```python
from build123d import *

# Parameters (mm, degrees)
SKETCH1_W           = 70
SKETCH1_H           = 25
SKETCH1_R           = 1.6
BOSS_EXTRUDE2_DEPTH = 10
SKETCH2_W           = 70
SKETCH2_H           = 5
BOSS_EXTRUDE3_DEPTH = 50
SKETCH3_R           = 3.5
CUT_EXTRUDE1_DEPTH  = 5
FILLET1_R           = 4
FILLET2_R           = 10
SKETCH4_R           = 1.6
CUT_EXTRUDE2_DEPTH  = 96.524865873


with BuildPart() as part:
    # Sketch1 → Boss-Extrude2 (new body)
    with BuildSketch(Plane(origin=(0, 0, 0), x_dir=(1, 0, 0), z_dir=(0, 1, 0))):
        with Locations((35, 12.5)):
            Rectangle(SKETCH1_W, SKETCH1_H)
        with Locations(Location((20, 15, 0), (0, 0, 270))):
            Circle(SKETCH1_R, mode=Mode.SUBTRACT)
        with Locations(Location((50, 15, 0), (0, 0, 270))):
            Circle(SKETCH1_R, mode=Mode.SUBTRACT)
    extrude(amount=BOSS_EXTRUDE2_DEPTH)

    # Sketch2 → Boss-Extrude3 (add)
    with BuildSketch(Plane(origin=(0, 10, 0), x_dir=(1, 0, 0), z_dir=(0, 1, 0))):
        with Locations((35, 2.5)):
            Rectangle(SKETCH2_W, SKETCH2_H)
    extrude(amount=BOSS_EXTRUDE3_DEPTH)

    # Sketch3 → Cut-Extrude1 (cut)
    with BuildSketch(Plane(origin=(0, 10, 0), x_dir=(1, 0, 0), z_dir=(0, 1, 0))):
        with Locations(Location((20, 15, 0), (0, 0, 270))):
            Circle(SKETCH3_R)
        with Locations(Location((50, 15, 0), (0, 0, 270))):
            Circle(SKETCH3_R)
    extrude(amount=-CUT_EXTRUDE1_DEPTH, mode=Mode.SUBTRACT)

    # Fillet1
    fillet1_edges = [part.edges().sort_by_distance(p)[0] for p in [
        (35, 10, -5),
    ]]
    fillet(fillet1_edges, radius=FILLET1_R)

    # Fillet2
    fillet2_edges = [part.edges().sort_by_distance(p)[0] for p in [
        (0, 60, -2.5),
        (70, 60, -2.5),
        (0, 5, -25),
        (70, 5, -25),
    ]]
    fillet(fillet2_edges, radius=FILLET2_R)

    # Sketch4 → Cut-Extrude2 (cut, through all)
    with BuildSketch(Plane.XY):
        with Locations((10, 50)):
            Circle(SKETCH4_R)
        with Locations((18, 50)):
            Circle(SKETCH4_R)
        with Locations((52, 50)):
            Circle(SKETCH4_R)
        with Locations((60, 50)):
            Circle(SKETCH4_R)
    extrude(amount=-CUT_EXTRUDE2_DEPTH, mode=Mode.SUBTRACT)


solid = part.part
```
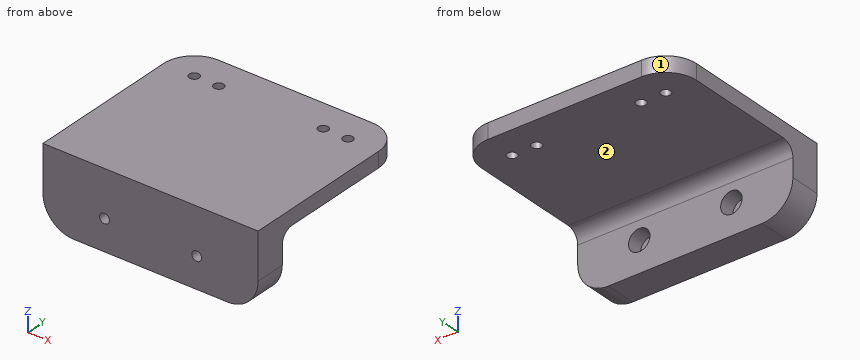
For this review, take the finished solid that the model builds, in its own axes (mm). Face numbers are marked on the shaded views. A direction names the side the tool comes from. Give positions to 0.01 mm unless a question says otherwise; leave off trailing zeros. Write each loop counter-clockwise with the first axis right and the second up, starting at its lowest first coordinate (ties: lowest second). Pieces come first, ordered by that corner, then holes.
Item 1: Wall thickness on probe 1 along X at (y, z) = (8.85, -15); probe 2 along X at (y, z) = (2.25, -15); probe 3 along Y at (x, z) = (10, -3.55): over which ranges is each line inside the solid? List them lowest first.
Item 2: Insertion check: P1, Ø5.5, axis at x = 19.5, z = -15.5, coming from the +Y side; P2, Ø3, axis at x = 33, y = 53, coming from the -Z side; P3, Ø8, axis at x = 24.5, z = -14.5, coming from the +Y side; P4, Ø10, axis at x = 62.5, z = -8, coming from the -Y side. Each pin has a flat end and moves straight along its axis. Give the tip position at first contact, or say it passes through.
Item 3: Take a section at A-A (x = 26). Give the boundary of the cut face in (y, z), and give its area (3 significant figures).
Item 4: Take a section at B-B (y = 42). Give the boundary of the cut face in (x, z).
Item 5: Machinability: for the marked faces 1 and 2, which of the approach directions +Z, -Z, +X, -X, +Y, -Y give a long, thin tool a straight path to every point of the face, cutting with its end or side? Answer none if there is none.
Established:
1. probe 1: x = 0 to 16.5, 23.5 to 46.5, 53.5 to 70
1. probe 2: x = 0 to 18.4, 21.6 to 48.4, 51.6 to 70
1. probe 3: y = 0 to 48.4, 51.6 to 60
2. P1: stops at y = 5
2. P2: stops at z = -5
2. P3: stops at y = 10
2. P4: stops at y = 0
3. outline: (0, -25) - (10, -25) - (10, -9) arc R4 cw to (14, -5) - (60, -5) - (60, 0) - (0, 0) - close
3. area: 503 mm2
4. outline: (0, -5) - (70, -5) - (70, 0) - (0, 0) - close
5. face 1: +Z, -Z, -X, +Y
5. face 2: -Z, +X, -X, +Y
